Part model, mm, in its own coordinate system. A direction names the side the tool comes from. Round coordinates to 2 decimals unless told otherwise and drop trailing zeros. Write each loop counter-clockwise with the first axis right and the second up, starting at its lowest first coordinate (ties: lowest second). Pieces come first, ordered by that corner, then holes. Notation, with made-up numbers: M 18,-31.5 L 65,-31.5 A18 ccw 65,-10.5 Z; hole C 22.25,54.25 d8. An arc over 180 degrees is marked long. Use one line per item in the form item = value. Start each with the question number.
Item 1: Which spindle directions (+Z, -Z, +X, -X, +Y, -Y) get a long thin tool onto all of the face, cutting with end or side? Do faces 4 (the face through (49, 3, -13.406)), 5 (the face through (1, 0, 0)), 6 (the face through (28, 5, 13)). Say none if no direction does.
Item 2: Cut at B-B, the plane z = 8.5. State how many separate pieces and enclosed holes the cut face has, then the cut area to 3 significant figures.
Item 3: Mould opens along Z. For faces 1 (the face through (0, 3, 30)), 2 (the face through (0, 3, -30)), 3 (the face through (34, 2, 10)) say: +Z half, -Z half, draft (parallel to the pull), parting line (faces both ways), or undercut.
Item 4: Cut at A-A, the plane x = -15. Give the cut face in (y, z), then the cut area to 3 significant figures.
Item 5: Flat gauge pins, fed straight in: pin 1 Ø2.5 at (x, z) = (33.5, -25) entering from -Y; pin 2 Ø4 at (x, y) = (47.5, 2) entering from +Z; pin 3 Ø5.5 at (x, y) = (50.5, 3) entering from -Z; pin 4 Ø1.5 at (y, z) = (5, 13.5) entering from +X. Where does each tip first touch, or does it go through?
Item 6: Probe L1, parallel to Z at x = 33.5, y = 3.7; L2, parallel to Y at x = -48, z = 6.5; L3, parallel to X at y = 2.25, z = 3. List the from-to ranges inside material, lowest first.
from build123d import *

# Parameters (mm, degrees)
BOSS_EXTRUDE1_DEPTH = 5
CUT_EXTRUDE1_DEPTH  = 71.407741052
BOSS_EXTRUDE2_DEPTH = 5
FILLET1_R           = 10
CUT_EXTRUDE2_DEPTH  = 71.938353519
M4_TAPPED_HOLE1_D   = 3.3
SKETCH13_W          = 2.5
SKETCH13_H          = 32.367781463
SKETCH17_W          = 2.5
SKETCH17_H          = 32.367781463
CHAMFER1_SIZE       = 3


with BuildPart() as part:
    # Sketch1 → Boss-Extrude1 (new body)
    with BuildSketch(Plane(origin=(0, 0, 0), x_dir=(1, 0, 0), z_dir=(0, 1, 0))):
        with BuildLine():
            Line((-33.5, 30), (33.5, 30))
            ThreePointArc((33.5, 30), (63.5, 0), (33.5, -30))
            Line((33.5, -30), (-33.5, -30))
            ThreePointArc((-33.5, -30), (-63.5, 0), (-33.5, 30))
        make_face()
        with BuildLine():
            Line((28.5, 10), (38.5, 10))
            ThreePointArc((38.5, 10), (48.5, 0), (38.5, -10))
            Line((38.5, -10), (28.5, -10))
            ThreePointArc((28.5, -10), (18.5, 0), (28.5, 10))
        make_face(mode=Mode.SUBTRACT)
    extrude(amount=BOSS_EXTRUDE1_DEPTH)

    # Sketch2 → Cut-Extrude1 (cut, through all)
    with BuildSketch(Plane(origin=(0, 5, 0), x_dir=(1, 0, 0), z_dir=(0, 1, 0))):
        with BuildLine():
            Line((13.943650814, 17.706349186), (21.943650814, 17.706349186))
            ThreePointArc((21.943650814, 17.706349186), (24.093650814, 15.556349186), (21.943650814, 13.406349186))
            Line((21.943650814, 13.406349186), (13.943650814, 13.406349186))
            ThreePointArc((13.943650814, 13.406349186), (11.793650814, 15.556349186), (13.943650814, 17.706349186))
        make_face()
        with BuildLine():
            Line((53.056349186, 17.706349186), (45.056349186, 17.706349186))
            ThreePointArc((45.056349186, 17.706349186), (42.906349186, 15.556349186), (45.056349186, 13.406349186))
            Line((45.056349186, 13.406349186), (53.056349186, 13.406349186))
            ThreePointArc((53.056349186, 13.406349186), (55.206349186, 15.556349186), (53.056349186, 17.706349186))
        make_face()
        with BuildLine():
            Line((53.056349186, -17.706349186), (45.056349186, -17.706349186))
            ThreePointArc((45.056349186, -17.706349186), (42.906349186, -15.556349186), (45.056349186, -13.406349186))
            Line((45.056349186, -13.406349186), (53.056349186, -13.406349186))
            ThreePointArc((53.056349186, -13.406349186), (55.206349186, -15.556349186), (53.056349186, -17.706349186))
        make_face()
        with BuildLine():
            Line((13.943650814, -17.706349186), (21.943650814, -17.706349186))
            ThreePointArc((21.943650814, -17.706349186), (24.093650814, -15.556349186), (21.943650814, -13.406349186))
            Line((21.943650814, -13.406349186), (13.943650814, -13.406349186))
            ThreePointArc((13.943650814, -13.406349186), (11.793650814, -15.556349186), (13.943650814, -17.706349186))
        make_face()
    extrude(amount=-CUT_EXTRUDE1_DEPTH, mode=Mode.SUBTRACT)

    # Sketch8 → Boss-Extrude2 (add)
    with BuildSketch(Plane(origin=(0, 5, 0), x_dir=(1, 0, 0), z_dir=(0, 1, 0))):
        with BuildLine():
            ThreePointArc((-33.5, -30), (-12.286796564, -21.213203436), (-3.5, 0))
            ThreePointArc((-3.5, 0), (-12.286796564, 21.213203436), (-33.5, 30))
            ThreePointArc((-33.5, 30), (-63.5, 0), (-33.5, -30))
        make_face()
        with BuildLine():
            Line((-3.5, 0), (-3.5, 30))
            Line((-3.5, 30), (-33.5, 30))
            ThreePointArc((-33.5, 30), (-12.286796564, 21.213203436), (-3.5, 0))
        make_face()
        with BuildLine():
            Line((-3.5, -30), (-3.5, 0))
            ThreePointArc((-3.5, 0), (-12.286796564, -21.213203436), (-33.5, -30))
            Line((-33.5, -30), (-3.5, -30))
        make_face()
    extrude(amount=BOSS_EXTRUDE2_DEPTH)

    # Fillet1
    # the kernel refuses this fillet: 10 mm, written as the material it adds along each edge
    with BuildSketch(Plane(origin=(-3.5, 5, -30), x_dir=(0, 1, 0), z_dir=(0, 0, 1))) as fillet1_piece_1:
        with BuildLine():
            CenterArc((10, -8.660254038), FILLET1_R, 120, 60)
            Line((0, -8.660254038), (-0.2, -8.660254038))
            Line((-0.2, -8.660254038), (-0.2, 0))
            Line((-0.2, 0), (0, 0.2))
            ThreePointArc((0, 0.2), (2.5, 0.2), (4.9, 0.173205081))
            Line((4.9, 0.173205081), (5, 0))
        make_face()
    extrude(amount=60)

    # Sketch9 → Cut-Extrude2 (cut, through all)
    with BuildSketch(Plane(origin=(0, 10, 0), x_dir=(1, 0, 0), z_dir=(0, 1, 0))):
        Polygon((-29.87232856, 9.966945366), (-23.533054634, -3.62767144), (-37.12767144, -9.966945366), (-43.466945366, 3.62767144), align=None)
    extrude(amount=-CUT_EXTRUDE2_DEPTH, mode=Mode.SUBTRACT)

    # M4 Tapped Hole1 (through all)
    with Locations(Plane(origin=(0, 5, 0), x_dir=(1, 0, 0), z_dir=(0, 1, 0))):
        with Locations((58.5, 0), (33.5, 25), (33.5, -25)):
            Hole(M4_TAPPED_HOLE1_D / 2)

    # Sketch13 → M6 Tapped Hole1 (revolve, cut)
    with BuildSketch(Plane(origin=(-40.297308403, 5, 3.169636963), x_dir=(-0.4226182617406973, 0, -0.9063077870366509), z_dir=(0, 1, 0))):
        with Locations((1.25, 16.183890732)):
            Rectangle(SKETCH13_W, SKETCH13_H)
    revolve(axis=Axis((-34.542253955, 5, 0.486011001), (-0.9063077870366509, 0, 0.42261826174069733)), mode=Mode.SUBTRACT)

    # Sketch17 → M6 Tapped Hole3 (revolve, cut)
    with BuildSketch(Plane(origin=(-36.669636963, 5, -6.797308403), x_dir=(0.9063077870366509, 0, -0.42261826174069766), z_dir=(0, 1, 0))):
        with Locations((1.25, 16.183890732)):
            Rectangle(SKETCH17_W, SKETCH17_H)
    revolve(axis=Axis((-33.986011001, 5, -1.042253955), (-0.42261826174069766, 0, -0.9063077870366508)), mode=Mode.SUBTRACT)

    # Chamfer1
    # the kernel refuses this chamfer: 3 mm, written as the material it takes off along each edge
    with BuildSketch(Plane(origin=(-33.5, 10, 30), x_dir=(0, 0.02749587661058619, -0.9996219169112968), z_dir=(1, 0, 0)), Plane(origin=(4.215048964, 10, -30), x_dir=(0, 0.02749587661058619, 0.9996219169112968), z_dir=(-1, 0, 0))) as chamfer1_piece_1:
        Polygon((CHAMFER1_SIZE * 0.999621916911, -CHAMFER1_SIZE * 0.0274958766106), (-CHAMFER1_SIZE * 0.0274958766106, -CHAMFER1_SIZE * 0.999621916911), (0, 0), align=None)
    extrude(amount=37.715048964, mode=Mode.SUBTRACT)
    with BuildSketch(Plane(origin=(-33.5, 10, 0), x_dir=(0, 0, 1), z_dir=(1, 0, 0))) as chamfer1_piece_2:
        Polygon((30 - CHAMFER1_SIZE, 0), (30, CHAMFER1_SIZE), (30, 0), align=None)
    revolve(axis=Axis((-33.5, 10, 0), (0, -1, 0)), revolution_arc=180, mode=Mode.SUBTRACT)


solid = part.part
Model answer:
q1.face_4 = +Y, -Y
q1.face_5 = +Z, -Z, +X, -X, -Y
q1.face_6 = +Z, -Z, +X, +Y
q2.separate_pieces = 3
q2.enclosed_holes = 1
q2.area = 737 mm²
q3.face_1 = +Z half
q3.face_2 = -Z half
q3.face_3 = undercut
q4.outline = M 0,-30 L 7,-30 L 10,-27 L 10,27 L 7,30 L 0,30 Z
q4.area = 591 mm²
q5.pin_1 = through
q5.pin_2 = 27.5
q5.pin_3 = -26.4
q5.pin_4 = 60.66
q6.L1 = -30 to -26.65, -23.35 to -10, 10 to 23.35, 26.65 to 30
q6.L2 = 0 to 2.51, 7.49 to 10
q6.L3 = -63.35 to -40.38, -23.83 to 18.96, 48.04 to 63.35
